The listing builds one solid part. Answer for the finished solid, in the listing's coordinates (mm). A direction names the side the tool comes from. Round coordinates to 2 decimals unless told otherwise and drop trailing zeros. Write each loop counter-clockwise with the first axis right and the second up, starting at its lowest first coordinate (ties: lowest second). Pieces come first, ordered by that corner, then holes. Notation, with made-up numbers: (-11.75, 54.5) - (46.25, 54.5) arc R11 cw to (46.25, 66.5) - close; hole circle Ø3 at (23, 79.5). An arc over 180 degrees is marked (long way). Return JSON: item names as keys, results as strings. Group by question number.
(1) Find the intervals of material crossed by line 1 along X through (y, z) = (-1.05, -0.55); line 2 along Y through (x, z) = (-1, 0.15); line 3 along Y through (x, z) = (5.5, 0.7), in increasing order. Write a range as [from, to].
(2) Section A-A, the plane x = 4 is taken. Write down the section's boundary in (y, z).
(3) Determine the mould class of faces 1 (the flat face through (8, 0, 0)), 2 (the flat face through (-1.5, 0.75, 0)), 3 (the cylindrical face through (4, 0, 1)) for opening direction Y: +Y half, -Y half, draft (parallel to the pull), parting line (faces both ways), or undercut.
(4) Each of these flat-tipped pins is pushed along its axis until it touches: pin 1 (2 mm diameter, centred on x = 5, y = 1.5, fed in from +Z); pin 2 (2 mm diameter, centred on x = 4, y = 0.5, fed in from -Z). Where does it stop, or does it pass through?
(5) Which of the six approach directions +Z, -Z, +X, -X, +Y, -Y give full straight-line access (tool end or side, diameter ignored) to faces 4 (the cylindrical face through (-0.91, -1.9, -0.08)), 5 (the flat face through (0, 1, -1)), 6 (the flat face through (-1.5, -0.75, 0))?
Autodesk Inventor part; units mm, degrees
ref_plane "Work Plane1" through (29, 0, 0) normal (0, -1, 0) x (1, 0, 0)
ref_plane "YZ Plane" through (0, 0, 0) normal (1, 0, 0) x (0, 1, 0)
ref_plane "XZ Plane" through (0, 0, 0) normal (0, 1, 0) x (-1, 0, 0)
sketch "Skizze1" plane through (0, 0, 0) normal (0, 0, 1) x (1, 0, 0)
  line L0 (-0.5, 0) -> (8, 0)
  line L1 (8, 0) -> (8, 1)
  line L2 (8, 1) -> (1.2, 1)
  line L3 (1.2, 1) -> (0.9545, 1)
  line L4 (0.9545, 1) -> (0, 1)
  line L5 (0, 1) -> (0, 1.9)
  line L6 (0, 1.9) -> (-2, 1.9)
  line L7 (-2, 1.9) -> (-2, 0.866)
  line L8 (-2, 0.866) -> (-1, 0.866)
  line L9 (-1, 0.866) -> (-0.5, 0)
  line L10 (-4, 0) -> (10, 0)
  line L11 (0, -0.38) -> (0, 2.28)
  line L12 (1.2, 1) -> (0, 1) construction
  dimension "d1" = 6.8
  dimension "d2" = 0.2455
  dimension "d3" = 2
  dimension "d4" = 1
  dimension "d5" = 60
  dimension "d6" = 2
  dimension "d7" = 2
  dimension "d8" = 1.7321
  dimension "d9" = 3.8
  dimension "d26" = 8
revolve "Körper" add sketch "Skizze1" angle 360 about axis through (-0.5, 0, 0) along (1, 0, 0)
sketch "Skizze2" plane through (-2, 0, 0) normal (-1, 0, 0) x (0, 0, 1)
  circle A0 centre (0, 0) radius 0.866
  line L0 (0, -2.66) -> (0, 2.66)
  line L1 (-2.66, 0) -> (2.66, 0)
  line L2 (0.866, 0) -> (0.433, -0.75)
  line L3 (0.433, -0.75) -> (-0.433, -0.75)
  line L4 (-0.433, -0.75) -> (-0.866, 0)
  line L5 (-0.866, 0) -> (-0.433, 0.75)
  line L6 (-0.433, 0.75) -> (0.433, 0.75)
  line L7 (0.433, 0.75) -> (0.866, 0)
  point P0 (0, 0)
extrude "Loch" add sketch "Skizze2" against normal up to next contours L7 A0 | A0 L2 | L6 L0 A0 | A0 L0 L3 | L0 L6 A0 | A0 L3 L0 | L4 A0 | A0 L5
fillet "Rundung1" radius 0.2 1 edges at (-2, -1.9, 0)
thread "Gewinde"
chamfer "Fase1" distance 0.2454 distance2 0.2454 1 edges at (8, -1, 0) measured on face at (8, 0.1182, 0.3117)
ref_plane "Work Plane1" through (29, 0, 0) normal (0, -1, 0) x (1, 0, 0)
fillet "Fillet2" radius 0.1 1 edges at (0, -1, 0)
equation "\"d1\" = GEL"
equation "\"d3\" = KOH"
equation "\"d4\" = INTI"
equation "\"d6\" = GD"
equation "\"d7\" = BDM"
equation "\"d8\" = 1.1547 * SW"
equation "\"d9\" = KOD"
equation "\"d26\" = NLG"
equation "\"d30\" = R"
equation "\"d17\" = RR"
equation "\"d13\" = GEL"
equation "\"d15\" = -0.5 * SPD + 0.5 * GD"
equation "\"d16\" = GUL"
equation "\"GD\" = 2"
equation "\"NLG\" = 8"
equation "\"GEL\" = 6.8"
equation "\"KOD\" = 3.8"
equation "\"KOH\" = 2"
equation "\"INTI\" = 1"
equation "\"GAL\" = 0.61345 * PTC"
equation "\"GUL\" = 0.61345 * PTC"
equation "\"BDM\" = NND"
equation "\"SW\" = 1.5"
equation "\"RR\" = 0.2"
equation "\"SPD\" = NND - 1.2269 * PTC"
equation "\"R\" = 0.1"
equation "\"TOA\" = 30deg"
equation "\"GD1\" = THREADDIA - 1.2269 * PTC"
equation "\"THREADDIA\" = 2"
equation "\"FAWI\" = 45deg"
equation "\"PTC\" = 0.4"
equation "\"NND\" = 2"
equation "\"E0\" = 1.155 * SW"
properties part number "ISO 4762  - M2 x 8" material "Edelstahl, 440C"
Working result:
{
 "1": {"line 1": "x = [-2, 0]", "line 2": "y = [-1.89, -0.75], [0.75, 1.89]", "line 3": "y = [-0.71, 0.71]"},
 "2": {"outline": "circle Ø2 at (0, 0)"},
 "3": {"face 1": "draft", "face 2": "undercut", "face 3": "parting line"},
 "4": {"pin 1": "stops at z = 0.87", "pin 2": "stops at z = -1"},
 "5": {"face 4": "+X, -X", "face 5": "+X", "face 6": "-X"}
}
